For this review, take the finished solid that the model builds, in its own axes (mm). Round coordinates to 2 decimals unless told otherwise and drop trailing zeros. Write each loop counter-clockwise with the first axis right and the second up, starting at its lowest first coordinate (ties: lowest second). Pieces come first, ordered by that corner, then holes.
from build123d import *

# Parameters (mm, degrees)
F0_W     = 229.429774
F0_H     = 125.460326
F1_DEPTH = 25.4
F2_R     = 10.16
F3_R     = 5.08


with BuildPart() as f1:
    # F0 (on Top) → F1 (new body)
    with BuildSketch(Plane.XY):
        with Locations((3.485013, -7.405646)):
            Rectangle(F0_W, F0_H)
    extrude(amount=F1_DEPTH)

    # F2
    f2_edges = [f1.edges().sort_by_distance(p)[0] for p in [
        (3.485013, 55.324517, 25.4),
        (-111.229874, -7.405646, 25.4),
        (3.485013, -70.135809, 25.4),
        (118.1999, -7.405646, 25.4),
    ]]
    fillet(f2_edges, radius=F2_R)

    # F3
    f3_edges = [f1.edges().sort_by_distance(p)[0] for p in [
        (3.485013, 55.324517, 0),
        (-111.229874, -7.405646, 0),
        (3.485013, -70.135809, 0),
        (118.1999, -7.405646, 0),
    ]]
    fillet(f3_edges, radius=F3_R)


solid = f1.part
(1) We need section A-A, the plane x = -19. Give the boundary of the cut face in (y, z).
Geometry check:
outline: (-70.14, 5.08) arc R5.08 ccw to (-65.06, 0) - (50.24, 0) arc R5.08 ccw to (55.32, 5.08) - (55.32, 15.24) arc R10.16 ccw to (45.16, 25.4) - (-59.98, 25.4) arc R10.16 ccw to (-70.14, 15.24) - close
(2) For line 1 along Y through (x, z) = (32, 20.5); line 2 along Y through (x, z) = (-83, 17.5); line 3 along X through (y, z) = (4.5, 4), list the stretches that pass through material, from the lowest coordinate up.
Geometry check:
line 1: y = -68.67 to 53.86
line 2: y = -69.88 to 55.07
line 3: x = -111.11 to 118.08
(3) For pin 1 Ø3 at (y, z) = (-6, 17.5) entering from -X; pin 2 Ø1.5 at (x, z) = (-15, 20.5) entering from -Y; pin 3 Ø4 at (x, z) = (-87.5, 18.5) entering from -Y, all flat-tipped, find the tip position at first contact; note any pin that passes through.
Geometry check:
pin 1: stops at x = -111.2
pin 2: stops at y = -69.08
pin 3: stops at y = -70.06
